Geometry check sheet. Reference: the model listing, model coordinates, mm. Round coordinates to 2 decimals unless told otherwise and drop trailing zeros. Loops run counter-clockwise (first coordinate to the right, second up) from the corner with the lowest first, then second, coordinate; pieces in that order, holes last. Notation, with made-up numbers: (64, 18) - (120, 18) arc R28 ccw to (120, 36) - close; hole circle Ø8 at (-39, 82.25). An arc over 180 degrees is marked (long way). Write item = value, one per line.
```python
from build123d import *

# Parameters (mm, degrees)
SKETCH1_W               = 202.4
SKETCH1_H               = 76.2
BOSS_EXTRUDE1_DEPTH     = 3
SKETCH2_R               = 7.5
CUT_EXTRUDE1_DEPTH      = 109.176013977
CUT_EXTRUDE2_DEPTH      = 109.176013977
CUT_EXTRUDE2_DEPTH_BACK = 109.176013977
SKETCH3_R               = 7.5


with BuildPart() as part:
    # Sketch1 → Boss-Extrude1 (new body)
    with BuildSketch(Plane.XY):
        Rectangle(SKETCH1_W, SKETCH1_H)
    extrude(amount=BOSS_EXTRUDE1_DEPTH)

    # Sketch2 → Cut-Extrude1 (cut, through all)
    with BuildSketch(Plane.XY.offset(3)):
        with Locations((-81.2, 0)):
            Circle(SKETCH2_R)
    extrude(amount=-CUT_EXTRUDE1_DEPTH, mode=Mode.SUBTRACT)

    # Sketch3 → Cut-Extrude2 (cut, two sides: drawn at the far end of the back side and taken through both)
    with BuildSketch(Plane.XY.offset(3).offset(-CUT_EXTRUDE2_DEPTH_BACK)):
        with Locations((-18.8, 0)):
            Circle(SKETCH3_R)
    extrude(amount=CUT_EXTRUDE2_DEPTH + CUT_EXTRUDE2_DEPTH_BACK, mode=Mode.SUBTRACT)


solid = part.part
```
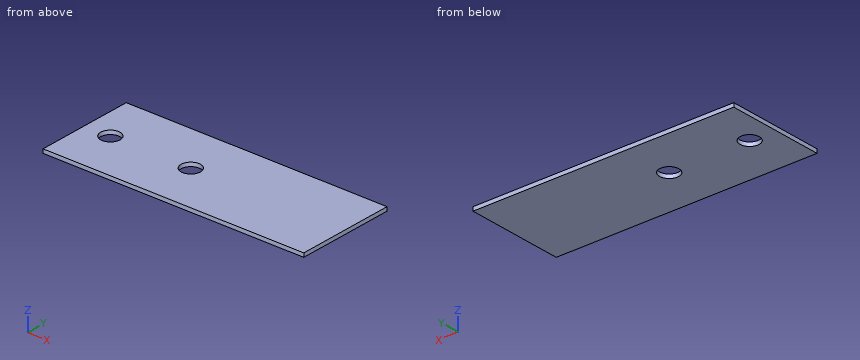
(1) Section check C-C (z = 1.95). Enter the section's corners in (x, y), then the cut area to 3 significant figures.
Answers follow:
outline = (-101.2, -38.1) - (101.2, -38.1) - (101.2, 38.1) - (-101.2, 38.1) - close; hole circle Ø15 at (-81.2, 0); hole circle Ø15 at (-18.8, 0)
area = 15,100 mm²
(2) Gauge pin test, flat end, axial feed: pin 1 (9 mm diameter, centred on x = -18.8, y = 0, fed in from +Z). Record the tip position at first contact, or that the pin passes through.
Answers follow:
pin_1 = through
(3) Section check A-A (y = 0). Enter the section's corners in (x, z).
Answers follow:
outline = (-101.2, 0) - (-88.7, 0) - (-88.7, 3) - (-101.2, 3) - close; (-73.7, 0) - (-26.3, 0) - (-26.3, 3) - (-73.7, 3) - close; (-11.3, 0) - (101.2, 0) - (101.2, 3) - (-11.3, 3) - close
(4) Section check B-B (x = -81.2). Enter the section's corners in (y, z), then the cut area to 3 significant figures.
Answers follow:
outline = (-38.1, 0) - (-7.5, 0) - (-7.5, 3) - (-38.1, 3) - close; (7.5, 0) - (38.1, 0) - (38.1, 3) - (7.5, 3) - close
area = 184 mm²
(5) Scan lines: L1, parallel to Y at x = -81.2, z = 1.45; L2, parallel to Y at x = -25.5, z = 2.35. Record each from-to range of solid material in increasing order. Write a range as [from, to].
Answers follow:
L1 = [-38.1, -7.5], [7.5, 38.1]
L2 = [-38.1, -3.37], [3.37, 38.1]
